CAD build for the part. Positions are in the model's coordinates, mm. A direction names the side the tool comes from. Round coordinates to 2 decimals unless told otherwise and drop trailing zeros. Write each loop counter-clockwise with the first axis right and the second up, starting at its lowest first coordinate (ties: lowest second). Pieces come first, ordered by that corner, then holes. Notation, with made-up numbers: (67, 20) - (118, 20) arc R13 ccw to (118, 31) - close; hole circle Ø3 at (-11.75, 7). An arc over 180 degrees is marked (long way). Put each result on its own line as item: value. Start each with the question number.
Item 1: Cut at A-A (y = 7). Give the cut face in (x, z), and give its area (3 significant figures).
Item 2: Mould opens along Y. For faces 1 (the flat face through (7.851, 4, -2)), 2 (the cylindrical face through (-7.02, 17.46, -3.39)), 3 (the flat face through (-2, 0, -2)) say: released by +Y, released by -Y, zero draft, split by the parting line, or undercut.
Item 3: Cut at B-B (z = 4.25). Count the separate pieces of the cut face and the enclosed holes in it, and give its area (3 significant figures).
Item 4: Cut at C-C (y = 13). Give the cut face in (x, z).
Item 5: Pin check, flat tips, straight feed: pin 1 Ø0.8 at (x, y) = (-1, 6.5) entering from +Z; pin 2 Ø6 at (y, z) = (18.5, 3) entering from -X; pin 3 Ø5 at (x, z) = (-1.5, -8.5) entering from +Y; pin 4 Ø2.5 at (x, z) = (-7, 3) entering from +Y. Stop position of each tip, or through.
Item 6: Drill centre lines: line 1 (Y direction, x = 3.25, z = -7.5); line 2 (Y direction, x = -5.75, z = -7.25); line 3 (X direction, y = 19.75, z = -6.75). Where is each one in solid material? Low to high. Write a range as from..to.
Item 7: 3-axis set-ups, long thin cutter, end or side, ignore diameter. For faces 4 (the flat face through (-7, 11, -8)), 5 (the cylindrical face through (-1.561, 6.268, -9.163)), 6 (the flat face through (4, 15, -3)), 7 (the flat face through (4, 11, -8)): which of +Z, -Z, +X, -X, +Y, -Y reach the whole face in a straight line?
```python
from build123d import *

# Parameters (mm, degrees)
SKETCH1_W           = 19
SKETCH1_H           = 19
BOSS_EXTRUDE1_DEPTH = 9
BOSS_EXTRUDE2_START = 9
SKETCH1_2_W         = 19
SKETCH1_2_H         = 19
BOSS_EXTRUDE2_DEPTH = 2
BOSS_EXTRUDE2_TAPER = 45
FILLET1_R           = 3
SKETCH2_R           = 7.5
BOSS_EXTRUDE3_DEPTH = 4
SKETCH3_R           = 5.5
BOSS_EXTRUDE4_DEPTH = 5
SKETCH4_R           = 8.5
BOSS_EXTRUDE5_DEPTH = 5.5
DOME1_FACE_RADIUS   = 8.5
DOME1_HEIGHT        = 1
SKETCH5_R           = 0.75
CUT_EXTRUDE1_DEPTH  = 5
CUT_EXTRUDE2_START  = -14
SKETCH5_2_R         = 0.75
CUT_EXTRUDE2_DEPTH  = 5


with BuildPart() as part:
    # Sketch1 → Boss-Extrude1 (new body)
    with BuildSketch(Plane(origin=(0, 0, 0), x_dir=(1, 0, 0), z_dir=(0, 1, 0))):
        with Locations((-1.648760331, 2.198347107)):
            Rectangle(SKETCH1_W, SKETCH1_H)
    extrude(amount=BOSS_EXTRUDE1_DEPTH)

    # Sketch1<2> → Boss-Extrude2 (add)
    with BuildSketch(Plane(origin=(0, 0, 0), x_dir=(1, 0, 0), z_dir=(0, 1, 0)).offset(BOSS_EXTRUDE2_START)):
        with Locations((-1.648760331, 2.198347107)):
            Rectangle(SKETCH1_2_W, SKETCH1_2_H)
    extrude(amount=BOSS_EXTRUDE2_DEPTH, taper=BOSS_EXTRUDE2_TAPER)

    # Fillet1
    fillet1_edges = [part.edges().sort_by_distance(p)[0] for p in [
        (6.851239669, 10, 6.301652893),
        (6.851239669, 10, -10.698347107),
        (-10.148760331, 10, -10.698347107),
        (-10.148760331, 10, 6.301652893),
    ]]
    fillet(fillet1_edges, radius=FILLET1_R)

    # Sketch2 → Boss-Extrude3 (add)
    with BuildSketch(Plane(origin=(0, 11, 0), x_dir=(1, 0, 0), z_dir=(0, 1, 0))):
        with Locations(Location((-1.648760331, 2.198347107, 0), (0, 0, 270))):
            Circle(SKETCH2_R)
    extrude(amount=BOSS_EXTRUDE3_DEPTH)

    # Sketch3 → Boss-Extrude4 (add)
    with BuildSketch(Plane(origin=(0, 15, 0), x_dir=(1, 0, 0), z_dir=(0, 1, 0))):
        with Locations(Location((-1.648760331, 2.198347107, 0), (0, 0, 270))):
            Circle(SKETCH3_R)
    extrude(amount=BOSS_EXTRUDE4_DEPTH)

    # Sketch4 → Boss-Extrude5 (add)
    with BuildSketch(Plane(origin=(0, 20, 0), x_dir=(1, 0, 0), z_dir=(0, 1, 0))):
        with Locations(Location((-1.648760331, 2.198347107, 0), (0, 0, 90))):
            Circle(SKETCH4_R)
    extrude(amount=BOSS_EXTRUDE5_DEPTH)

    # Dome1: a dome of height H over a round flat face of radius A is a cap of a sphere of radius (A * A + H * H) / (2 * H)
    dome1_r = (DOME1_FACE_RADIUS * DOME1_FACE_RADIUS + DOME1_HEIGHT * DOME1_HEIGHT) / (2 * DOME1_HEIGHT)
    dome1_base = Plane((-1.648760331, 25.5, -2.198347107), z_dir=(0, 1, 0))
    with Locations(dome1_base.offset(DOME1_HEIGHT - dome1_r)):
        dome1_ball = Sphere(dome1_r, mode=Mode.PRIVATE)
    add(split(dome1_ball, bisect_by=dome1_base, keep=Keep.TOP, mode=Mode.PRIVATE))

    # Sketch5 → Cut-Extrude1 (cut)
    with BuildSketch(Plane.XY.offset(7.301652893)):
        with Locations((-1.398760331, 7)):
            Circle(SKETCH5_R)
    extrude(amount=-CUT_EXTRUDE1_DEPTH, mode=Mode.SUBTRACT)

    # Sketch5<2> → Cut-Extrude2 (cut)
    with BuildSketch(Plane.XY.offset(7.301652893).offset(CUT_EXTRUDE2_START)):
        with Locations((-1.398760331, 7)):
            Circle(SKETCH5_2_R)
    extrude(amount=-CUT_EXTRUDE2_DEPTH, mode=Mode.SUBTRACT)


solid = part.part
```
Output values:
1. outline: (-11.15, -11.7) - (-2.15, -11.7) - (-2.15, -6.7) - (-0.65, -6.7) - (-0.65, -11.7) - (7.85, -11.7) - (7.85, 7.3) - (-0.65, 7.3) - (-0.65, 2.3) - (-2.15, 2.3) - (-2.15, 7.3) - (-11.15, 7.3) - close
1. area: 346 mm2
2. face 1: zero draft
2. face 2: undercut
2. face 3: released by -Y
3. separate pieces: 2
3. enclosed holes: 1
3. area: 298 mm2
4. outline: circle Ø15 at (-1.65, -2.2)
5. pin 1: z = 7.3
5. pin 2: x = -9.74
5. pin 3: y = 26.3
5. pin 4: y = 25.97
6. line 1: 0..15, 20..25.78
6. line 2: 0..15, 20..25.92
6. line 3: -4.74..1.44
7. face 4: -Z, -X
7. face 5: -Z
7. face 6: none
7. face 7: -Z, +X
